```python
from build123d import *

# Parameters (mm, degrees)
ESQUISSE1_R             = 6
BOSS_EXTRU_1_DEPTH      = 50
ENL_V_MAT_EXTRU_3_DEPTH = 2
BOSS_EXTRU_2_START      = 15
ESQUISSE4_R             = 6
BOSS_EXTRU_2_DEPTH      = 15


with BuildPart() as part:
    # Esquisse1 → Boss.-Extru.1 (new body)
    with BuildSketch(Plane.XY):
        Circle(ESQUISSE1_R)
    extrude(amount=-BOSS_EXTRU_1_DEPTH)

    # Esquisse3 → Enlèv. mat.-Extru.3 (cut)
    with BuildSketch(Plane(origin=(0, 6, 0), x_dir=(1, 0, 0), z_dir=(0, 1, 0))):
        with BuildLine():
            Line((2, 39), (2, 28))
            ThreePointArc((2, 28), (0, 26), (-2, 28))
            Line((-2, 28), (-2, 39))
            ThreePointArc((-2, 39), (0, 41), (2, 39))
        make_face()
    extrude(amount=-ENL_V_MAT_EXTRU_3_DEPTH, mode=Mode.SUBTRACT)

    # Esquisse4 → Boss.-Extru.2 (add)
    with BuildSketch(Plane.XY.offset(BOSS_EXTRU_2_START)):
        Circle(ESQUISSE4_R)
    extrude(amount=-BOSS_EXTRU_2_DEPTH)


solid = part.part
```
Check sheet for the modelled part. Datum: model origin and axes. Units: mm. A direction names the side the tool comes from. Coordinates: 2 decimals unless noted, no trailing zeros. Order: outer loops, then holes, each group sorted by start corner. A loop starts at its lowest first (then second) coordinate and runs counter-clockwise, first axis right, second up. Notation, with made-up numbers: (86.5, -6) -> (109.5, -6) arc R9 ccw to (109.5, 9) -> close; hole circle Ø6 at (75.5, 86.5). An arc over 180 degrees is marked (long way). Write each question's results on one line, items separated by ' | '. Start each with the question number.
1) Section check C-C (z = -38). Enter the section's corners in (x, y).
2) Depth check by flat-ended pin: pin 1 (2 mm diameter, centred on y = 4.5, z = -12, fed in from +X); pin 2 (0.5 mm diameter, centred on y = 5, z = -33.5, fed in from -X); pin 3 (1.5 mm diameter, centred on x = -1.5, z = -21.5, fed in from +Y). Enter the tip coordinate at first touch or a pass-through.
3) Section check D-D (y = -5). Enter the section's corners in (x, z), and give its area (3 significant figures).
4) Section check B-B (y = 5). Enter the section's corners in (x, z), and give its area (3 significant figures).
5) Draft check along Z on faces 1 (the face through (-1.301, -5.857, -17.045)), 2 (the face through (0, 0, 15)), 3 (the face through (0, 5, -41)). Enter one of: pulls with the +Z half, pulls with the -Z half, needs draft (parallel to the pull), parting line crosses it, or undercut.
6) Section check A-A (x = 0). Enter the section's corners in (y, z).
7) Set-up check for faces 4 (the face through (0, 0, -50)), 5 (the face through (-2, 5, -33)): record each of +Z, -Z, +X, -X, +Y, -Y from which the full face is reachable in a straight line by a thin tool's end or side.
8) Material ranges on line 1 along Y through (x, z) = (-0.25, -30); line 2 along X through (y, z) = (-0.25, 2.5); line 3 along Y through (x, z) = (-2.25, -19), recorded low to high.
Checked values:
1) outline: (-2, 4) -> (-2, 5.66) arc R6 ccw (long way) to (2, 5.66) -> (2, 4) -> close
2) pin 1: x = 4.87 | pin 2: x = -3.67 | pin 3: y = 5.95
3) outline: (-3.32, -50) -> (3.32, -50) -> (3.32, 15) -> (-3.32, 15) -> close | area: 431 mm²
4) outline: (-3.32, -50) -> (3.32, -50) -> (3.32, 15) -> (-3.32, 15) -> close; hole (-2, -39) arc R2 ccw to (2, -39) -> (2, -28) arc R2 ccw to (-2, -28) -> close | area: 375 mm²
5) face 1: needs draft | face 2: pulls with the +Z half | face 3: undercut
6) outline: (-6, -50) -> (6, -50) -> (6, -41) -> (4, -41) -> (4, -26) -> (6, -26) -> (6, 15) -> (-6, 15) -> close
7) face 4: -Z, +X, -X, +Y, -Y | face 5: +Y
8) line 1: -5.99 to 4 | line 2: -5.99 to 5.99 | line 3: -5.56 to 5.56
